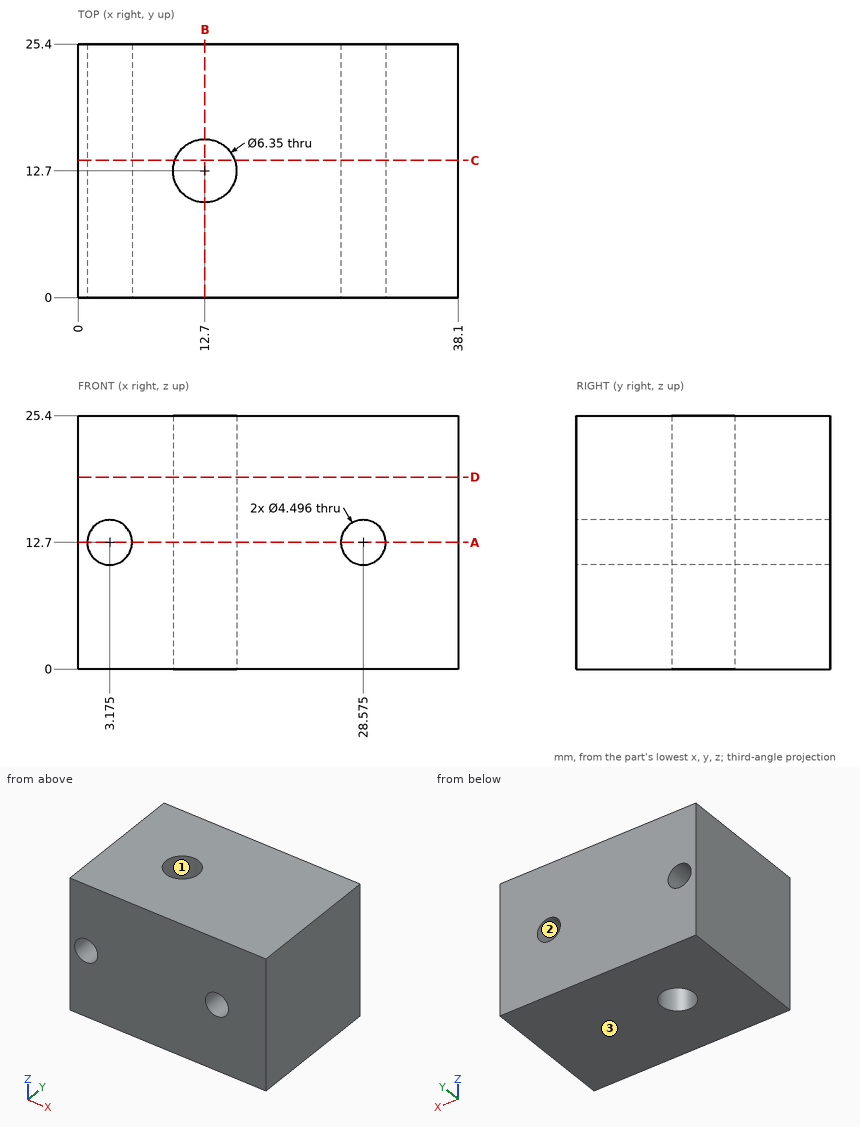
Input: dimensioned drawing with shaded views. Units: mm. Origin: part minimum x, y, z. Coordinates: 2 decimals unless noted, no trailing zeros. Loops run counter-clockwise (first coordinate to the right, second up) from the corner with the lowest first, then second, coordinate; pieces in that order, holes last.
Q1. Line query: line 1 along X through (y, z) = (13, 14); line 2 along X through (y, z) = (12.7, 18.25) (3 decimals); line 3 along X through (y, z) = (14.5, 12.7) (1 decimal). Output: solid intervals per line, ascending.
Results are:
line 1: x = 0 to 1.34, 5.01 to 9.54, 15.86 to 26.74, 30.41 to 38.1
line 2: x = 0 to 9.525, 15.875 to 38.1
line 3: x = 0 to 0.9, 5.4 to 10.1, 15.3 to 26.3, 30.8 to 38.1
Q2. Section C-C, the plane y = 13.75. Return the cut outline in (x, z) (1 decimal).
Results are:
outline: (0, 0) - (9.7, 0) - (9.7, 25.4) - (0, 25.4) - close; (15.7, 0) - (38.1, 0) - (38.1, 25.4) - (15.7, 25.4) - close; hole circle Ø4.5 at (3.2, 12.7); hole circle Ø4.5 at (28.6, 12.7)
Q3. Mould query, pull axis Z, two halves, no side actions, for the marked faces 1, 2 and 3. Classes: +Z half, -Z half, draft (parallel to the pull), parting line (faces both ways), or undercut.
Results are:
face 1: draft
face 2: undercut
face 3: -Z half
Q4. Contact query for a flat-ended pin moving along its axis: pin 1 (2.5 mm diameter, centred on x = 3.175, z = 12.7, fed in from -Y). Output: stop coordinate, or through.
Results are:
pin 1: passes through
Q5. Section A-A, the plane z = 12.7. Give the number of separate pieces and of enclosed holes in the cut face, and give its area (3 significant figures).
Results are:
separate pieces: 3
enclosed holes: 1
area: 708 mm2
Q6. Section D-D, the plane z = 19.25. Return the cut outline in (x, y) (3 decimals), and give its area (3 significant figures).
Results are:
outline: (0, 0) - (38.1, 0) - (38.1, 25.4) - (0, 25.4) - close; hole circle Ø6.35 at (12.7, 12.7)
area: 936 mm2
Q7. Section B-B, the plane x = 12.7. Return the cut outline in (y, z) (3 decimals), and give its area (3 significant figures).
Results are:
outline: (0, 0) - (9.525, 0) - (9.525, 25.4) - (0, 25.4) - close; (15.875, 0) - (25.4, 0) - (25.4, 25.4) - (15.875, 25.4) - close
area: 484 mm2
